Build history of the part. All positions in model axes, mm. A direction names the side the tool comes from. Give positions to 0.01 mm unless a question says otherwise; leave off trailing zeros. Write each loop counter-clockwise with the first axis right and the second up, starting at its lowest first coordinate (ties: lowest second). Pieces come first, ordered by that corner, then holes.
from build123d import *

# Parameters (mm, degrees)
SKETCH_1_R        = 19
SKETCH_1_R_2      = 13
SKETCH_1_R_3      = 1.25
EXTRUDE_1_DEPTH   = 5
SKETCH_2_R        = 14.5
SKETCH_2_R_2      = 13
EXTRUDE_1_2_DEPTH = 15.5
SKETCH_3_R        = 14.5
SKETCH_3_R_2      = 13
SKETCH_3_R_3      = 7
SKETCH_3_R_4      = 1.5
EXTRUDE_2_DEPTH   = 2


with BuildPart() as part:
    # 草图1 → Extrude 1 (new body)
    with BuildSketch(Plane(origin=(0, 0, 0), x_dir=(1, 0, 0), z_dir=(0, 1, 0))):
        with Locations(Location((0, 0, 0), (0, 0, 270))):
            Circle(SKETCH_1_R)
        with Locations(Location((0, 0, 0), (0, 0, 270))):
            Circle(SKETCH_1_R_2, mode=Mode.SUBTRACT)
        with Locations(Location((0, 17, 0), (0, 0, 270))):
            Circle(SKETCH_1_R_3, mode=Mode.SUBTRACT)
        with Locations(Location((14.722431864, -8.5, 0), (0, 0, 270))):
            Circle(SKETCH_1_R_3, mode=Mode.SUBTRACT)
        with Locations(Location((-14.722431864, -8.5, 0), (0, 0, 270))):
            Circle(SKETCH_1_R_3, mode=Mode.SUBTRACT)
    extrude(amount=EXTRUDE_1_DEPTH)

    # 草图2 → Extrude 1 2 (add)
    with BuildSketch(Plane(origin=(0, 5, 0), x_dir=(1, 0, 0), z_dir=(0, 1, 0))):
        Circle(SKETCH_2_R)
        Circle(SKETCH_2_R_2, mode=Mode.SUBTRACT)
    extrude(amount=EXTRUDE_1_2_DEPTH)

    # 草图3 → 凸台-拉伸2 (add)
    # profile 1 of 2: a face of its own
    with BuildSketch(Plane(origin=(0, 20.5, 0), x_dir=(1, 0, 0), z_dir=(0, 1, 0))):
        Circle(SKETCH_3_R)
        with Locations(Location((0, 0, 0), (0, 0, 270))):
            Circle(SKETCH_3_R_2, mode=Mode.SUBTRACT)
    # profile 2 of 2: a face of its own
    with BuildSketch(Plane(origin=(0, 20.5, 0), x_dir=(1, 0, 0), z_dir=(0, 1, 0))):
        with Locations(Location((0, 0, 0), (0, 0, 270))):
            Circle(SKETCH_3_R_2)
        with Locations(Location((0, 0, 0), (0, 0, 270))):
            Circle(SKETCH_3_R_3, mode=Mode.SUBTRACT)
        with Locations(Location((-7.27742221, 6.106482292, 0), (0, 0, 270))):
            Circle(SKETCH_3_R_4, mode=Mode.SUBTRACT)
        with Locations(Location((-8.927079897, -3.249191362, 0), (0, 0, 270))):
            Circle(SKETCH_3_R_4, mode=Mode.SUBTRACT)
        with Locations(Location((-1.649657688, -9.355673654, 0), (0, 0, 270))):
            Circle(SKETCH_3_R_4, mode=Mode.SUBTRACT)
        with Locations(Location((7.27742221, -6.106482292, 0), (0, 0, 270))):
            Circle(SKETCH_3_R_4, mode=Mode.SUBTRACT)
        with Locations(Location((8.927079897, 3.249191362, 0), (0, 0, 270))):
            Circle(SKETCH_3_R_4, mode=Mode.SUBTRACT)
        with Locations(Location((1.649657688, 9.355673654, 0), (0, 0, 270))):
            Circle(SKETCH_3_R_4, mode=Mode.SUBTRACT)
    extrude(amount=EXTRUDE_2_DEPTH)


solid = part.part
1. Saw through at A-A on z = -17. Give the cut face in (x, y), plus the area to 3 significant figures.
2. 3-axis set-ups, long thin cutter, end or side, ignore diameter. For faces 1 (the face through (-6, 20.5, 6)), 2 (the face through (-7, 5, -13)), 3 (the face through (2.1, 21.486, -7.925)): which of +Z, -Z, +X, -X, +Y, -Y reach the whole face in a straight line?
3. Saw through at B-B on y = 21. Give the cut face in (x, z), plus the area to 3 significant figures.
4. Mould opens along X. For faces 4 (the face through (4.5, 0, 12.4)), 5 (the face through (6.691, 13.628, 12.864)), 6 (the face through (13.96, 2.46, 7.51)) say: pulls with the +X half, pulls with the -X half, needs draft (parallel to the pull), parting line crosses it, or undercut.
5. Drop flat-ended pins along their axis: pin 1 (5 mm diameter, centred on x = 2.5, z = -5.5, fed in from -Y); pin 2 (1 mm diameter, centred on x = 8.5, y = 8.5, fed in from +Z); pin 3 (2.5 mm diameter, centred on x = -8.93, z = 3.25, fed in from +Y); pin 4 (10 mm diameter, centred on y = 12, z = 0, fed in from +X). Give the stop position or say it passes through.
6. Drill centre lines: line 1 along X through (y, z) = (1.2, 8.5); line 2 along X through (y, z) = (20.75, -3); line 3 along Z through (x, y) = (-1, 2). Where is each one in solid material? Low to high.
7. Saw through at D-D on y = 3.75. Give the cut face in (x, z), plus the area to 3 significant figures.
Outcome:
1. outline: (-8.49, 0) - (-1.25, 0) - (-1.25, 5) - (-8.49, 5) - close; (1.25, 0) - (8.49, 0) - (8.49, 5) - (1.25, 5) - close
1. area: 72.4 mm2
2. face 1: -Y
2. face 2: +Y
2. face 3: +Y, -Y
3. outline: circle Ø29 at (0, 0); hole circle Ø3 at (-8.93, 3.25); hole circle Ø3 at (-7.28, -6.11); hole circle Ø14 at (0, 0); hole circle Ø3 at (-1.65, 9.36); hole circle Ø3 at (1.65, -9.36); hole circle Ø3 at (7.28, 6.11); hole circle Ø3 at (8.93, -3.25)
3. area: 464 mm2
4. face 4: needs draft
4. face 5: parting line crosses it
4. face 6: undercut
5. pin 1: stops at y = 20.5
5. pin 2: stops at z = 12.09
5. pin 3: passes through
5. pin 4: stops at x = 14.5
6. line 1: x = -16.99 to -15.97, -13.47 to -9.84, 9.84 to 13.47, 15.97 to 16.99
6. line 2: x = -14.19 to -6.32, 6.32 to 7.45, 10.41 to 14.19
6. line 3: z = -18.97 to -17.75, -16.25 to -12.96, 12.96 to 18.97
7. outline: circle Ø38 at (0, 0); hole circle Ø2.5 at (-14.72, 8.5); hole circle Ø26 at (0, 0); hole circle Ø2.5 at (0, -17); hole circle Ø2.5 at (14.72, 8.5)
7. area: 588 mm2
